```python
from build123d import *

# Parameters (mm, degrees)
BOSS_EXTRUDE1_DEPTH = 165


with BuildPart() as part:
    # Sketch1 → Boss-Extrude1 (new body)
    with BuildSketch(Plane(origin=(0, 0, -65), x_dir=(-1, 0, 0), z_dir=(0, 0, -1))):
        with BuildLine():
            Line((-14.999999999, 12.999999999), (-14.999999999, 10.499999999))
            Line((-14.999999999, 10.499999999), (-14.499999999, 9.999999999))
            Line((-14.499999999, 9.999999999), (-14.999999999, 9.5))
            Line((-14.999999999, 9.5), (-14.999999999, 4.5))
            Line((-14.999999999, 4.5), (-14.5, 4.5))
            Line((-14.5, 4.5), (-14.5, 4))
            Line((-14.5, 4), (-12.200000005, 4))
            Line((-12.200000005, 4), (-12.200000005, 7.999999995))
            ThreePointArc((-12.200000005, 7.999999995), (-11.582683434, 8.923879532), (-10.492893215, 8.70710678))
            Line((-10.492893215, 8.70710678), (-6, 4.214213564))
            Line((-6, 4.214213564), (-6, 0.312520903))
            Line((-6, 0.312520903), (-5.7, 0))
            Line((-5.7, 0), (-6, -0.312520901))
            Line((-6, -0.312520901), (-6, -4.214213564))
            Line((-6, -4.214213564), (-10.492893215, -8.70710678))
            ThreePointArc((-10.492893215, -8.70710678), (-11.582683434, -8.923879532), (-12.200000005, -7.999999995))
            Line((-12.200000005, -7.999999995), (-12.200000005, -4))
            Line((-12.200000005, -4), (-14.5, -4))
            Line((-14.5, -4), (-14.5, -4.5))
            Line((-14.5, -4.5), (-14.999999999, -4.5))
            Line((-14.999999999, -4.5), (-14.999999999, -9.500000003))
            Line((-14.999999999, -9.500000003), (-14.499999999, -10.000000002))
            Line((-14.499999999, -10.000000002), (-14.999999999, -10.500000001))
            Line((-14.999999999, -10.500000001), (-14.999999999, -13))
            ThreePointArc((-14.999999999, -13), (-14.414213561, -14.414213562), (-12.999999999, -15))
            Line((-12.999999999, -15), (-10.5, -15))
            Line((-10.5, -15), (-10.000000001, -14.500000001))
            Line((-10.000000001, -14.500000001), (-9.500000001, -15))
            Line((-9.500000001, -15), (-4.5, -15))
            Line((-4.5, -15), (-4.5, -14.5))
            Line((-4.5, -14.5), (-4, -14.5))
            Line((-4, -14.5), (-4, -12.200000005))
            Line((-4, -12.200000005), (-7.999999995, -12.200000005))
            ThreePointArc((-7.999999995, -12.200000005), (-8.923879532, -11.582683434), (-8.70710678, -10.492893215))
            Line((-8.70710678, -10.492893215), (-4.214213564, -6))
            Line((-4.214213564, -6), (-0.312520903, -6))
            Line((-0.312520903, -6), (0, -5.7))
            Line((0, -5.7), (0.312520901, -6))
            Line((0.312520901, -6), (4.214213564, -6))
            Line((4.214213564, -6), (8.70710678, -10.492893215))
            ThreePointArc((8.70710678, -10.492893215), (8.923879532, -11.582683434), (7.999999995, -12.200000005))
            Line((7.999999995, -12.200000005), (4, -12.200000005))
            Line((4, -12.200000005), (4, -14.5))
            Line((4, -14.5), (4.5, -14.5))
            Line((4.5, -14.5), (4.5, -15))
            Line((4.5, -15), (9.500000001, -15))
            Line((9.500000001, -15), (9.989897949, -14.5))
            Line((9.989897949, -14.5), (10.489897949, -15))
            Line((10.489897949, -15), (13, -15))
            ThreePointArc((13, -15), (14.414213562, -14.414213562), (15, -13))
            Line((15, -13), (15, -10.5))
            Line((15, -10.5), (14.500000001, -10.000000001))
            Line((14.500000001, -10.000000001), (15, -9.500000001))
            Line((15, -9.500000001), (15, -4.5))
            Line((15, -4.5), (14.5, -4.5))
            Line((14.5, -4.5), (14.5, -4))
            Line((14.5, -4), (12.200000005, -4))
            Line((12.200000005, -4), (12.200000005, -7.999999995))
            ThreePointArc((12.200000005, -7.999999995), (11.582683434, -8.923879532), (10.492893215, -8.70710678))
            Line((10.492893215, -8.70710678), (6, -4.214213564))
            Line((6, -4.214213564), (6, -0.312520903))
            Line((6, -0.312520903), (5.7, 0))
            Line((5.7, 0), (6, 0.312520901))
            Line((6, 0.312520901), (6, 4.214213564))
            Line((6, 4.214213564), (10.492893215, 8.707106779))
            ThreePointArc((10.492893215, 8.707106779), (11.582683434, 8.923879532), (12.200000005, 7.999999994))
            Line((12.200000005, 7.999999994), (12.200000005, 4))
            Line((12.200000005, 4), (14.5, 4))
            Line((14.5, 4), (14.5, 4.5))
            Line((14.5, 4.5), (15, 4.5))
            Line((15, 4.5), (15, 9.500000001))
            Line((15, 9.500000001), (14.500000001, 10.000000001))
            Line((14.500000001, 10.000000001), (15, 10.5))
            Line((15, 10.5), (15, 12.999999999))
            ThreePointArc((15, 12.999999999), (14.414213562, 14.414213561), (13, 14.999999999))
            Line((13, 14.999999999), (10.500000001, 14.999999999))
            Line((10.500000001, 14.999999999), (10.000000002, 14.499999999))
            Line((10.000000002, 14.499999999), (9.500000003, 14.999999999))
            Line((9.500000003, 14.999999999), (4.5, 14.999999999))
            Line((4.5, 14.999999999), (4.5, 14.5))
            Line((4.5, 14.5), (4, 14.5))
            Line((4, 14.5), (4, 12.200000005))
            Line((4, 12.200000005), (7.999999995, 12.200000005))
            ThreePointArc((7.999999995, 12.200000005), (8.923879532, 11.582683434), (8.70710678, 10.492893215))
            Line((8.70710678, 10.492893215), (4.214213564, 6))
            Line((4.214213564, 6), (0.312520903, 6))
            Line((0.312520903, 6), (0, 5.7))
            Line((0, 5.7), (-0.312520901, 6))
            Line((-0.312520901, 6), (-4.214213564, 6))
            Line((-4.214213564, 6), (-8.707106779, 10.492893215))
            ThreePointArc((-8.707106779, 10.492893215), (-8.923879532, 11.582683434), (-7.999999994, 12.200000005))
            Line((-7.999999994, 12.200000005), (-4, 12.200000005))
            Line((-4, 12.200000005), (-4, 14.5))
            Line((-4, 14.5), (-4.5, 14.5))
            Line((-4.5, 14.5), (-4.5, 14.999999999))
            Line((-4.5, 14.999999999), (-9.5, 14.999999999))
            Line((-9.5, 14.999999999), (-9.999999999, 14.499999999))
            Line((-9.999999999, 14.499999999), (-10.499999999, 14.999999999))
            Line((-10.499999999, 14.999999999), (-12.999999999, 14.999999999))
            ThreePointArc((-12.999999999, 14.999999999), (-14.414213561, 14.414213561), (-14.999999999, 12.999999999))
        make_face()
        with BuildLine():
            Line((4.808326112, 3.676955262), (2.902349714, 1.770978864))
            ThreePointArc((2.902349714, 1.770978864), (3.4, 0), (2.902349714, -1.770978864))
            Line((2.902349714, -1.770978864), (4.808326112, -3.676955262))
            Line((4.808326112, -3.676955262), (3.676955262, -4.808326112))
            Line((3.676955262, -4.808326112), (1.770978864, -2.902349714))
            ThreePointArc((1.770978864, -2.902349714), (0, -3.4), (-1.770978864, -2.902349714))
            Line((-1.770978864, -2.902349714), (-3.676955262, -4.808326112))
            Line((-3.676955262, -4.808326112), (-4.808326112, -3.676955262))
            Line((-4.808326112, -3.676955262), (-2.902349714, -1.770978864))
            ThreePointArc((-2.902349714, -1.770978864), (-3.4, 0), (-2.902349714, 1.770978864))
            Line((-2.902349714, 1.770978864), (-4.808326112, 3.676955262))
            Line((-4.808326112, 3.676955262), (-3.676955262, 4.808326112))
            Line((-3.676955262, 4.808326112), (-1.770978864, 2.902349714))
            ThreePointArc((-1.770978864, 2.902349714), (0, 3.4), (1.770978864, 2.902349714))
            Line((1.770978864, 2.902349714), (3.676955262, 4.808326112))
            Line((3.676955262, 4.808326112), (4.808326112, 3.676955262))
        make_face(mode=Mode.SUBTRACT)
    extrude(amount=-BOSS_EXTRUDE1_DEPTH)


solid = part.part
```
Can you work these out from the model? Positions are in its coordinate system, mm. A direction names the side the tool comes from. Coordinates: 2 decimals unless noted, no trailing zeros. Put each result on its own line as item: value. Start each with the question number.
Q1. If I drill on line 1 (X direction, y = 10.5, z = -42); line 2 (X direction, y = -5, z = 57); line 3 (Y direction, x = -3.5, z = 39.5), over which ranges is the centre line in solid material (lowest first)? Write a range as [from, to].
Q2. Thinking about a two-plate mould opening in X: for faces 3 (the face through (-8.215, 6.429, 16.345)), 4 (the face through (-7, 15, 16)), 5 (the face through (15, -7, 16)), which applies, pulls with the +X half, pulls with the -X half, needs draft (parallel to the pull), parting line crosses it, or undercut?
Q3. I'm going to push flat-ended pins straight in: P1, Ø1.8, axis at y = -14, z = 54.5, coming from the -X side; P2, Ø4, axis at x = 0.5, z = -13.5, coming from the +Y side; P3, Ø1.8, axis at x = -14, z = 2.5, coming from the +Y side; P4, Ø1.5, axis at x = -11, y = 6.5, coming from the -Z side. Where does each tip first touch, or does it pass through?
Q4. For faces 1 (the face through (7, 15, 16)), 2 (the face through (3.4, 0, 16.3)), which set-ups out of +Z, -Z, +X, -X, +Y, -Y let a thin tool reach every point of the face, with its end or its side?
Taken from the geometry:
1. line 1: x = [-15, -8.71], [8.71, 15]
1. line 2: x = [-15, -12.2], [-6.79, 6.79], [12.2, 15]
1. line 3: y = [-6, -4.63], [-2.37, 2.37], [4.63, 6]
2. face 3: undercut
2. face 4: needs draft
2. face 5: pulls with the +X half
3. P1: stops at x = -15
3. P2: stops at y = 6
3. P3: stops at y = 15
3. P4: passes through
4. face 1: +Z, -Z, +X, -X, +Y
4. face 2: +Z, -Z
